```python
from build123d import *

# Parameters (mm, degrees)
SKETCH1_R           = 6.5
SKETCH1_R_2         = 7.5
BOSS_EXTRUDE1_DEPTH = 10


with BuildPart() as part:
    # Sketch1 → Boss-Extrude1 (new body)
    with BuildSketch(Plane.XY):
        with BuildLine():
            Line((-90, 25), (-90, 15))
            Line((-90, 15), (-61, 7.769487918))
            Line((-61, 7.769487918), (-61, -7.769487918))
            Line((-61, -7.769487918), (-90, -15))
            Line((-90, -15), (-90, -25))
            Line((-90, -25), (-49, -25))
            Line((-49, -25), (-44.767984939, -9.205904774))
            ThreePointArc((-44.767984939, -9.205904774), (-42.982162953, -6.533233299), (-39.938355808, -5.5))
            Line((-39.938355808, -5.5), (-18.186533479, -5.5))
            ThreePointArc((-18.186533479, -5.5), (0, -19), (18.186533479, -5.5))
            Line((18.186533479, -5.5), (49.907414279, -5.5))
            ThreePointArc((49.907414279, -5.5), (53.789878627, -7.349369811), (54.800298032, -11.529411765))
            ThreePointArc((54.800298032, -11.529411765), (52.301289102, -20.014373791), (48.497422612, -28))
            ThreePointArc((48.497422612, -28), (53.255752861, -45.758330249), (71.01408311, -41))
            ThreePointArc((71.01408311, -41), (82, 0), (71.01408311, 41))
            ThreePointArc((71.01408311, 41), (53.255752861, 45.758330249), (48.497422612, 28))
            ThreePointArc((48.497422612, 28), (52.301289102, 20.014373791), (54.800298032, 11.529411765))
            ThreePointArc((54.800298032, 11.529411765), (53.789878627, 7.349369811), (49.907414279, 5.5))
            Line((49.907414279, 5.5), (18.186533479, 5.5))
            ThreePointArc((18.186533479, 5.5), (0, 19), (-18.186533479, 5.5))
            Line((-18.186533479, 5.5), (-39.938355808, 5.5))
            ThreePointArc((-39.938355808, 5.5), (-42.982162953, 6.533233299), (-44.767984939, 9.205904774))
            Line((-44.767984939, 9.205904774), (-49, 25))
            Line((-49, 25), (-90, 25))
        make_face()
        Circle(SKETCH1_R, mode=Mode.SUBTRACT)
        with Locations((59.755752861, 34.5)):
            Circle(SKETCH1_R_2, mode=Mode.SUBTRACT)
        with Locations((59.755752861, -34.5)):
            Circle(SKETCH1_R_2, mode=Mode.SUBTRACT)
    extrude(amount=BOSS_EXTRUDE1_DEPTH)


solid = part.part
```
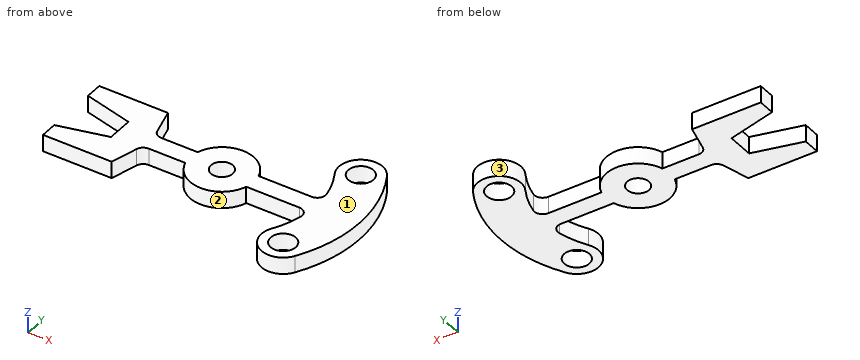
For this review, take the finished solid that the model builds, in its own axes (mm). Face numbers are marked on the shaded views. Coordinates: 2 decimals unless noted, no trailing zeros. Write each loop counter-clockwise with the first axis right and the second up, starting at its lowest first coordinate (ties: lowest second). Pieces come first, ordered by that corner, then holes. Notation, with made-up numbers: (-19, 65.5) - (-12, 65.5) arc R8 cw to (-12, 79.5) - close; hole circle Ø2 at (-13.75, -37.5). An arc over 180 degrees is marked (long way). Answer in a Markdown table with one row per item. Add a question column.
Q1. We need section D-D, the plane x = 28. State the section outline as (y, z) points, and give its area (3 significant figures).
Q2. We need section B-B, the plane y = 0. State the section outline as (x, z) points, and give its area (3 significant figures).
Q3. For probe 1 along X at (y, z) = (0.5, 9.25); probe 2 along Y at (x, z) = (-25.5, 3); probe 3 along Y at (x, z) = (-62, 0.75), list the stretches that pass through material, from the lowest coordinate up.
Q4. We need section C-C, the plane z = 2.25. State the section outline as (x, y) points, and give its area (3 significant figures).
Q5. For P1, Ø3, axis at y = 8, z = 1.5, coming from the +X side; P2, Ø4, axis at x = -55, z = 3, coming from the +Y side; P3, Ø9, axis at x = 59.76, y = 34.5, coming from the +Z side (1 decimal); P4, Ø5, axis at x = 33, z = 4, coming from the +Y side, all flat-tipped, find the tip position at first contact; note any pin that passes through.
Q6. Draft analysis for pull direction X (two halves, no side actions). For the marked faces 1, 2 and 3, state which applies: +X half, -X half, draft (parallel to the pull), parting line (faces both ways), or undercut.
Q7. We need section A-A, the plane x = 0. State the section outline as (y, z) points.
Answer list:
| question | item | result |
|---|---|---|
| 1 | outline | (-5.5, 0) - (5.5, 0) - (5.5, 10) - (-5.5, 10) - close |
| 1 | area | 110 mm2 |
| 2 | outline | (-61, 0) - (-6.5, 0) - (-6.5, 10) - (-61, 10) - close; (6.5, 0) - (82, 0) - (82, 10) - (6.5, 10) - close |
| 2 | area | 1,300 mm2 |
| 3 | probe 1 | x = -61 to -6.48, 6.48 to 82 |
| 3 | probe 2 | y = -5.5 to 5.5 |
| 3 | probe 3 | y = -25 to -8.02, 8.02 to 25 |
| 4 | outline | (-90, -25) - (-49, -25) - (-44.77, -9.21) arc R5 cw to (-39.94, -5.5) - (-18.19, -5.5) arc R19 ccw to (18.19, -5.5) - (49.91, -5.5) arc R5 cw to (54.8, -11.53) arc R56 cw to (48.5, -28) arc R13 ccw to (71.01, -41) arc R82 ccw to (71.01, 41) arc R13 ccw to (48.5, 28) arc R56 cw to (54.8, 11.53) arc R5 cw to (49.91, 5.5) - (18.19, 5.5) arc R19 ccw to (-18.19, 5.5) - (-39.94, 5.5) arc R5 cw to (-44.77, 9.21) - (-49, 25) - (-90, 25) - (-90, 15) - (-61, 7.77) - (-61, -7.77) - (-90, -15) - close; hole circle Ø13 at (0, 0); hole circle Ø15 at (59.76, -34.5); hole circle Ø15 at (59.76, 34.5) |
| 4 | area | 5,310 mm2 |
| 5 | P1 | stops at x = 81.74 |
| 5 | P2 | stops at y = 25 |
| 5 | P3 | passes through |
| 5 | P4 | stops at y = 5.5 |
| 6 | face 1 | draft |
| 6 | face 2 | undercut |
| 6 | face 3 | parting line |
| 7 | outline | (-19, 0) - (-6.5, 0) - (-6.5, 10) - (-19, 10) - close; (6.5, 0) - (19, 0) - (19, 10) - (6.5, 10) - close |
